The listing builds one solid part. Answer for the finished solid, in the listing's coordinates (mm). A direction names the side the tool comes from. Coordinates: 2 decimals unless noted, no trailing zeros. Loops run counter-clockwise (first coordinate to the right, second up) from the corner with the lowest first, then second, coordinate; pieces in that order, holes last. Notation, with made-up numbers: (72, -40) - (107, -40) arc R16 cw to (107, -18) - close; hole circle Ø8 at (18.5, -2). An arc over 180 degrees is marked (long way). One line per question, with ' | ' between items.
from build123d import *

# Parameters (mm, degrees)
F1_DEPTH = 1473.939
F3_DEPTH = 254.001
F5_DEPTH = 6.35


with BuildPart() as f1:
    # F0 (on Front) → F1 (new body)
    with BuildSketch(Plane.XZ):
        with BuildLine():
            Line((-41.275, 0), (-9.525, 0))
            ThreePointArc((-9.525, 0), (-2.789808, 2.789808), (0, 9.525))
            Line((0, 9.525), (0, 244.475))
            ThreePointArc((0, 244.475), (-2.789808, 251.210192), (-9.525, 254))
            Line((-9.525, 254), (-41.275, 254))
            ThreePointArc((-41.275, 254), (-48.010192, 251.210192), (-50.8, 244.475))
            Line((-50.8, 244.475), (-50.8, 9.525))
            ThreePointArc((-50.8, 9.525), (-48.010192, 2.789808), (-41.275, 0))
        make_face()
        with BuildLine():
            ThreePointArc((-46.0502, 244.5004), (-44.659016, 247.859016), (-41.3004, 249.2502))
            Line((-41.3004, 249.2502), (-9.4996, 249.2502))
            ThreePointArc((-9.4996, 249.2502), (-6.140984, 247.859016), (-4.7498, 244.5004))
            Line((-4.7498, 244.5004), (-4.7498, 9.4996))
            ThreePointArc((-4.7498, 9.4996), (-6.140984, 6.140984), (-9.4996, 4.7498))
            Line((-9.4996, 4.7498), (-41.3004, 4.7498))
            ThreePointArc((-41.3004, 4.7498), (-44.659016, 6.140984), (-46.0502, 9.4996))
            Line((-46.0502, 9.4996), (-46.0502, 244.5004))
        make_face(mode=Mode.SUBTRACT)
    extrude(amount=F1_DEPTH)

    # F2 (on face) → F3 (cut, through all)
    with BuildSketch(Plane.XY.offset(254)):
        Polygon((0, -1423.139), (-50.8, -1473.939), (0, -1473.939), align=None)
        Polygon((0, 0), (-50.8, 0), (0, -50.8), align=None)
    extrude(amount=-F3_DEPTH, mode=Mode.SUBTRACT)


with BuildPart() as f5:
    # F4 (on face) → F5 (new body)
    with BuildSketch(Plane.YZ):
        with BuildLine():
            ThreePointArc((-262.900179, 386.417484), (-267.477327, 385.56399), (-271.439268, 383.118226))
            Line((-271.439268, 383.118226), (-298.414744, 358.615267))
            ThreePointArc((-298.414744, 358.615267), (-301.488932, 354.354737), (-302.575654, 349.214525))
            Line((-302.575654, 349.214525), (-302.575654, 238.994726))
            ThreePointArc((-302.575654, 238.994726), (-298.85591, 230.01447), (-289.875654, 226.294726))
            Line((-289.875654, 226.294726), (-220.098802, 226.294726))
            ThreePointArc((-220.098802, 226.294726), (-211.118546, 230.01447), (-207.398802, 238.994726))
            Line((-207.398802, 238.994726), (-207.398802, 373.717484))
            ThreePointArc((-207.398802, 373.717484), (-211.118546, 382.69774), (-220.098802, 386.417484))
            Line((-220.098802, 386.417484), (-262.900179, 386.417484))
        make_face()
    extrude(amount=F5_DEPTH)


with BuildPart() as f6_1:
    # F6: copy of F5
    add(f5.part)


solid = f1.part
Item 1: The mould has two halves that part along Z. Classify faces 1 (the face through (-25, -727, 254)), 2 (the face through (-25, -727, 4.75)), 3 (the face through (0, -727, 125)): pulls with the +Z half, pulls with the -Z half, needs draft (parallel to the pull), parting line crosses it, or undercut.
Taken from the geometry:
face 1: pulls with the +Z half | face 2: undercut | face 3: needs draft
Item 2: Find section C-C, the plane y = -1237. Write down the section's boundary in (x, z) (3 decimals).
Taken from the geometry:
outline: (-50.8, 9.525) arc R9.525 ccw to (-41.275, 0) - (-9.525, 0) arc R9.525 ccw to (0, 9.525) - (0, 244.475) arc R9.525 ccw to (-9.525, 254) - (-41.275, 254) arc R9.525 ccw to (-50.8, 244.475) - close; hole (-46.05, 9.5) arc R4.75 ccw to (-41.3, 4.75) - (-9.5, 4.75) arc R4.75 ccw to (-4.75, 9.5) - (-4.75, 244.5) arc R4.75 ccw to (-9.5, 249.25) - (-41.3, 249.25) arc R4.75 ccw to (-46.05, 244.5) - close
Item 3: Find the intervals of material crossed by line 1 (X direction, y = -748, z = 35); line 2 (Z direction, x = -18, y = -1188.5); line 3 (Z direction, x = -43.5, y = -1289), in increasing order. Write a range as [from, to].
Taken from the geometry:
line 1: x = [-50.8, -46.05], [-4.75, 0] | line 2: z = [0, 4.75], [249.25, 254] | line 3: z = [0.26, 5.29], [248.71, 253.74]
Item 4: Find section A-A, the plane z = 220. Write down the section's boundary in (x, y), plus the area to 3 significant figures.
Taken from the geometry:
outline: (-50.8, -1473.94) - (-46.05, -1469.19) - (-46.05, -4.75) - (-50.8, 0) - close; (-4.75, -1427.89) - (0, -1423.14) - (0, -50.8) - (-4.75, -46.05) - close | area: 13,500 mm2
Item 5: Which of the six approach directions +Z, -Z, +X, -X, +Y, -Y give full straight-line access (tool end or side, diameter ignored) to faces 4 (the face through (-46.2, -4.6, 137)), 5 (the face through (-46.05, -727, 125))?
Taken from the geometry:
face 4: +Z, -Z, +X, +Y | face 5: +Y, -Y
Item 6: Find section B-B, the plane x = -31.5. Write down the section's boundary in (y, z).
Taken from the geometry:
outline: (-1454.64, 0) - (-19.3, 0) - (-19.3, 4.75) - (-1454.64, 4.75) - close; (-1454.64, 249.25) - (-19.3, 249.25) - (-19.3, 254) - (-1454.64, 254) - close
